```python
from build123d import *

# Parameters (mm, degrees)
F0_W     = 25
F0_H     = 3.598708484
F0_H_2   = 2.5
F0_H_3   = 44.7172746155
F0_W_2   = 6
F0_H_4   = 35
F1_DEPTH = 3
F2_DEPTH = 10
F3_START = 10
F3_DEPTH = 3
F4_R     = 4
F5_R     = 3


# Not quite as in the source:
# - a feature names something its author has since deleted; it is built from what else it names


with BuildPart() as f1:
    # F0 (on Top) → F1 (new body)
    with BuildSketch(Plane.XY):
        with Locations((0.1855289564, 2.9724632242)):
            Rectangle(F0_W, F0_H)
        with Locations((0.1855289564, -0.0768910178)):
            Rectangle(F0_W, F0_H_2)
        with Locations((0.1855289564, 27.130454774)):
            Rectangle(F0_W, F0_H_3)
        with Locations((-6.4080492333, 27.7351317182)):
            Rectangle(F0_W_2, F0_H_4, mode=Mode.SUBTRACT)
        with Locations((6.5919507667, 27.7351317182)):
            Rectangle(F0_W_2, F0_H_4, mode=Mode.SUBTRACT)
    extrude(amount=F1_DEPTH)

    # F0 (on Top) → F2 (join)
    with BuildSketch(Plane.XY):
        with Locations((0.1855289564, -0.0768910178)):
            Rectangle(F0_W, F0_H_2)
    extrude(amount=F2_DEPTH)

    # F0 (on Top) → F3 (join)
    with BuildSketch(Plane.XY.offset(F3_START)):
        with Locations((0.1855289564, 2.9724632242)):
            Rectangle(F0_W, F0_H)
        Polygon((-12.3144710436, -1.3268910178), (-12.3144710436, 1.1731089822), (-12.3144710436, 4.7718174662), (-15.4697376937, 4.7718174662), (-15.4697376937, -5.2281825338), (16.5302623063, -5.2281825338), (16.5302623063, 4.7718174662), (12.6855289564, 4.7718174662), (12.6855289564, 1.1731089822), (12.6855289564, -1.3268910178), align=None)
        with Locations((0.1855289564, -0.0768910178)):
            Rectangle(F0_W, F0_H_2)
    extrude(amount=F3_DEPTH)

    # F4
    f4_edges = [f1.edges().sort_by_distance(p)[0] for p in [
        (16.530262, -5.228183, 11.5),
        (16.530262, 4.771817, 11.5),
        (-15.469738, -5.228183, 11.5),
        (-15.469738, 4.771817, 11.5),
    ]]
    fillet(f4_edges, radius=F4_R)

    # F5
    f5_edges = [f1.edges().sort_by_distance(p)[0] for p in [
        (-12.314471, 49.489092, 1.5),
        (12.685529, 49.489092, 1.5),
    ]]
    fillet(f5_edges, radius=F5_R)


solid = f1.part
```
Geometry: final body of the model. Coordinates: model frame, mm. A direction names the side the tool comes from. Coordinates: 2 decimals unless noted, no trailing zeros. Loops run counter-clockwise (first coordinate to the right, second up) from the corner with the lowest first, then second, coordinate; pieces in that order, holes last. Notation, with made-up numbers: M 23,45.25 L 66,45.25 A27 cw 66,74.25 Z; hole C 7.25,15.5 d10. An arc over 180 degrees is marked long. Put each result on its own line as item: value.
(1) Cut plane B-B on x = -8.5. Return the cut outline in (y, z), then the cut area to 3 significant figures.
Answer sheet:
outline: M -5.23,10 L -1.33,10 L -1.33,0 L 10.24,0 L 10.24,3 L 1.17,3 L 1.17,10 L 4.77,10 L 4.77,13 L -5.23,13 Z; M 45.24,0 L 49.49,0 L 49.49,3 L 45.24,3 Z
area: 94.9 mm^2
(2) Cut plane A-A on y = 33. Return the cut outline in (x, z), then the cut area to 3 significant figures.
Answer sheet:
outline: M -12.31,0 L -9.41,0 L -9.41,3 L -12.31,3 Z; M -3.41,0 L 3.59,0 L 3.59,3 L -3.41,3 Z; M 9.59,0 L 12.69,0 L 12.69,3 L 9.59,3 Z
area: 39.0 mm^2
(3) Cut plane C-C on z = 1.25. Return the cut outline in (x, y), then the cut area to 3 significant figures.
Answer sheet:
outline: M -12.31,-1.33 L 12.69,-1.33 L 12.69,46.49 A3 ccw 9.69,49.49 L -9.31,49.49 A3 ccw -12.31,46.49 Z; hole M -9.41,10.24 L -3.41,10.24 L -3.41,45.24 L -9.41,45.24 Z; hole M 3.59,10.24 L 9.59,10.24 L 9.59,45.24 L 3.59,45.24 Z
area: 847 mm^2
(4) Material intervals for probe 1 along X at (y, z) = (24.5, 2.75); probe 2 along Z at (x, y) = (-9, 2.5); probe 3 along Y at (x, z) = (9, 1.5), sorted ascending.
Answer sheet:
probe 1: x = -12.31 to -9.41, -3.41 to 3.59, 9.59 to 12.69
probe 2: z = 0 to 3, 10 to 13
probe 3: y = -1.33 to 10.24, 45.24 to 49.49
(5) Access query for faces 4 (the face through (-9.408, 27, 1)), 5 (the face through (12.686, 16.9, 2.7)), 6 (the face through (0, -1.327, 5)). Directions: +Z, -Z, +X, -X, +Y, -Y. A direction counts if a zero-diameter tool reaches every point of the face in a straight line with its end or side. Return the directions, or none.
Answer sheet:
face 4: +Z, -Z
face 5: -Z, +X, +Y, -Y
face 6: -Z, +X, -X, -Y
(6) Draft query along Y for faces 1 (the face through (-6, 10.235, 1)), 2 (the face through (0, 24, 0)), 3 (the face through (-11.459, 48.587, 1.521)). Return one class per face: pulls with the +Y half, pulls with the -Y half, needs draft (parallel to the pull), parting line crosses it, or undercut.
Answer sheet:
face 1: undercut
face 2: needs draft
face 3: pulls with the +Y half
(7) First-contact query: pin 1 (0.9 mm diameter, centred on x = -4, z = 12, fed in from +Y); pin 2 (3.5 mm diameter, centred on x = 7, z = 1, fed in from -Y); pin 3 (5 mm diameter, centred on x = 0, z = 7, fed in from +Y). Flat tips, straight axial feed; report the tip coordinate or a pass-through.
Answer sheet:
pin 1: stops at y = 4.77
pin 2: stops at y = -1.33
pin 3: stops at y = 1.17
(8) Cut plane D-D on x = 3. Return the cut outline in (y, z), then the cut area to 3 significant figures.
Answer sheet:
outline: M -5.23,10 L -1.33,10 L -1.33,0 L 49.49,0 L 49.49,3 L 1.17,3 L 1.17,10 L 4.77,10 L 4.77,13 L -5.23,13 Z
area: 200 mm^2
